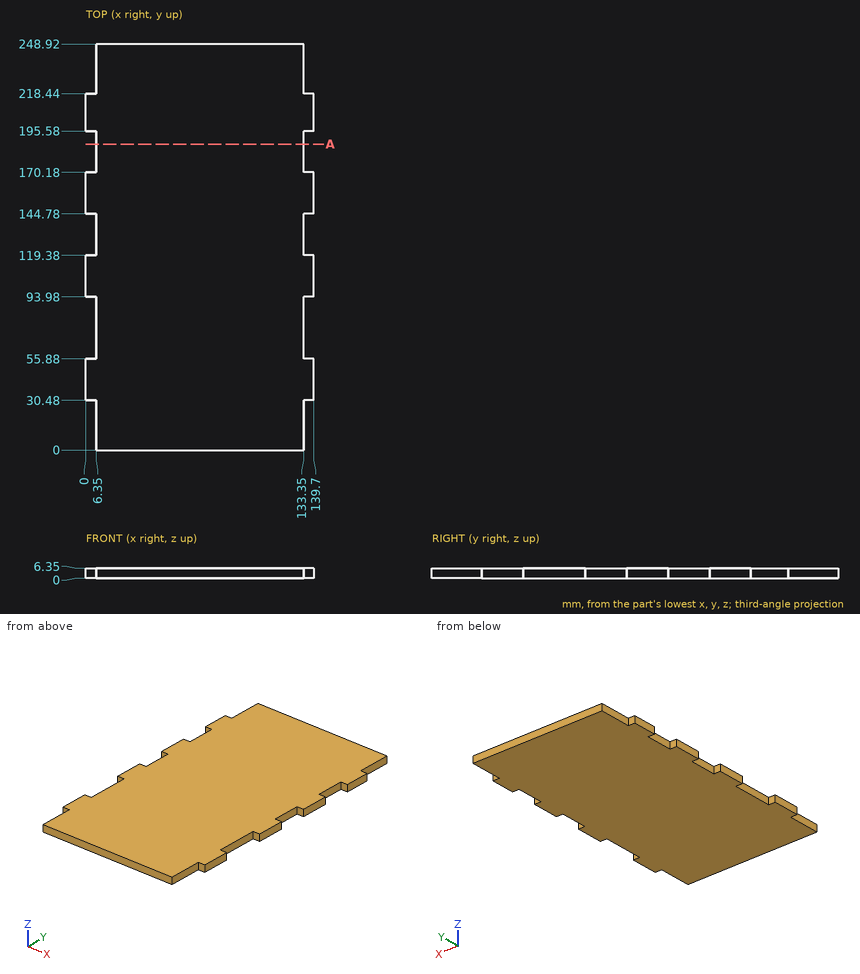
Could you check a few things on this drawing? It's one solid part, dimensions in mm from its lowest x, y, z. Give positions to 0.01 mm unless a question says otherwise; leave off trailing zeros. Order: outer loops, then holes, each group sorted by start corner. A loop starts at its lowest first (then second) coordinate and runs counter-clockwise, first axis right, second up. Notation, with made-up numbers: (25.25, 11.5) -> (44.25, 11.5) arc R7 cw to (44.25, 23.5) -> close; hole circle Ø10 at (30.25, 18.25). An arc over 180 degrees is marked (long way). Answer in a Markdown table with one row per item. Add a question column.
Item 1: I'm going to push flat-ended pins straight in: P1, Ø3, axis at x = 135.5, z = 4, coming from the -Y side; P2, Ø1.9, axis at x = 137, z = 4, coming from the +Y side; P3, Ø12, axis at x = 90, y = 132, coming from the -Z side; P4, Ø1.9, axis at y = 177, z = 3.5, coming from the +X side. Where does each tip first touch, or does it pass through?
Item 2: Imagine slicing it at A-A (y = 187.5). List the corners of the cut face in (x, z) for me, and give its area (3 significant figures).
Item 3: Please list where this line runs through material, in increasing order: probe 1 along X at (y, z) = (56.5, 1.25).
Result:
| question | item | result |
|---|---|---|
| 1 | P1 | y = 30.48 |
| 1 | P2 | y = 218.44 |
| 1 | P3 | z = 0 |
| 1 | P4 | x = 133.35 |
| 2 | outline | (6.35, 0) -> (133.35, 0) -> (133.35, 6.35) -> (6.35, 6.35) -> close |
| 2 | area | 806 mm2 |
| 3 | probe 1 | 6.35 to 133.35 |
